Source: CAD feature listing. Evaluate the final solid. Frame: model axes, mm. Face numbers are marked on the shaded views. A direction names the side the tool comes from. Give positions to 0.01 mm unless a question says otherwise; leave off trailing zeros. Order: outer loops, then holes, each group sorted by start corner. A loop starts at its lowest first (then second) coordinate and runs counter-clockwise, first axis right, second up. Notation, with made-up numbers: M 84.25,-21.5 L 130.25,-21.5 A22 cw 130.25,4.5 Z; hole C 73,70.25 d11. An arc over 180 degrees is marked long. Return JSON: item names as keys, results as strings.
Solid Edge part; units mm, degrees
sketch "Sketch1" plane through (0, 0, 0) normal (0, -1, 0) x (1, 0, 0)
  arc A0 (87.9904, -3.3394) -> (81.4545, -9.3797) centre (75, 4.1606) cw
  arc A1 (81.4545, -9.3797) -> (51.8166, -19.1606) centre (28.049, 102.6551) cw
  line L0 (-51.8166, -19.1606) -> (51.8166, -19.1606)
  arc A2 (-81.4545, -9.3797) -> (-51.8166, -19.1606) centre (-28.049, 102.6551) ccw
  arc A3 (-73.8916, 19.1195) -> (-81.4545, -9.3797) centre (-75, 4.1606) ccw
  arc A4 (73.8916, 19.1195) -> (-73.8916, 19.1195) centre (0, 1016.3858) cw
  arc A5 (73.8916, 19.1195) -> (89.9997, 4.062) centre (75, 4.1606) cw
  arc A6 (87.9904, -3.3394) -> (89.9997, 4.062) centre (75, 4.1606) ccw
extrude "Protrusion1" add sketch "Sketch1" along normal mid plane 10
sketch "Sketch2" plane through (0, 0, 0) normal (0, -1, 0) x (1, 0, 0)
  circle A0 centre (-75, 4.1606) radius 12.5
  circle A1 centre (-38.1427, -9.4726) radius 7.5
  circle A2 centre (-13.3438, -9.4726) radius 7.5
  circle A3 centre (13.3438, -9.4726) radius 7.5
  circle A4 centre (38.1427, -9.4726) radius 7.5
  circle A5 centre (75, 4.1606) radius 12.5
extrude "ExtrudedProtrusion_2" add sketch "Sketch2" along normal blind 10
sketch "Sketch3" plane through (-75, -10, 4.1606) normal (0, -1, 0) x (1, 0, 0)
  arc A0 (162.5, 0) -> (137.5, 0) centre (150, 0) ccw
  line L0 (12.5, 0) -> (137.5, 0)
  arc A1 (-12.5, 0) -> (12.5, 0) centre (0, 0) cw
  line L1 (-12.5, 0) -> (-18.0005, 0)
  line L2 (-18.0005, 0) -> (-4.7328, 20)
  line L3 (0, 20) -> (-4.7328, 20)
  line L4 (150, 20) -> (0, 20)
  line L5 (150, 20) -> (154.7328, 20)
  line L6 (168.0005, 0) -> (154.7328, 20)
  line L7 (162.5, 0) -> (168.0005, 0)
extrude "Protrusion2" add sketch "Sketch3" against normal up to vertex (15 mm away)
sketch "Sketch4" plane through (-75, -10, 4.1606) normal (0, -1, 0) x (1, 0, 0)
  line L0 (0, 0) -> (150, 0)
  line L1 (150, 0) -> (168.0005, 0)
  line L2 (168.0005, 0) -> (154.7328, 20)
  line L3 (150, 20) -> (154.7328, 20)
  line L4 (150, 20) -> (0, 20)
  line L5 (0, 20) -> (-4.7328, 20)
  line L6 (-18.0005, 0) -> (-4.7328, 20)
  line L7 (0, 0) -> (-18.0005, 0)
extrude "ExtrudedCutout_2" cut sketch "Sketch4" against normal blind 2
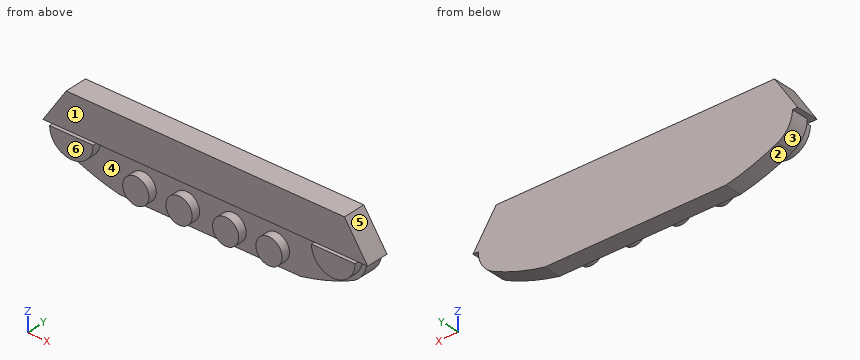
1. First-contact query: pin 1 (0.6 mm diameter, centred on x = -73.5, y = -8.5, fed in from +Z); pin 2 (8 mm diameter, centred on x = -42.5, z = 1.5, fed in from -Y); pin 3 (4.5 mm diameter, centred on x = 89.5, y = -1, fed in from -Z). Flat tips, straight axial feed; report the tip coordinate or a pass-through.
Evaluation:
{"pin 1": "stops at z = 4.16", "pin 2": "stops at y = -8", "pin 3": "stops at z = -4.5"}
2. Set-up query: the marked faces 1 and 2. Return all of +Z, -Z, +X, -X, +Y, -Y with unobstructed straight access to the full face (end or side cutting, diameter ignored); none if empty.
Evaluation:
{"face 1": "+Z, +X, -X, -Y", "face 2": "-Z, -X, +Y, -Y"}
3. Draft query along X for the marked faces 3, 4, 5 and 6. Return one class per face: pulls with the +X half, pulls with the -X half, needs draft (parallel to the pull), parting line crosses it, or undercut.
Evaluation:
{"face 3": "pulls with the -X half", "face 4": "undercut", "face 5": "pulls with the +X half", "face 6": "needs draft"}
4. Section query D-D (x = -74). Return loops of the section in (y, z), then the cut area to 3 significant figures.
Evaluation:
{"outline": "M -10,-8.3 L -5,-8.3 L -5,-12.64 L 5,-12.64 L 5,24.16 L -8,24.16 L -8,4.16 L -10,4.16 Z", "area": "490 mm^2"}
5. Section query B-B (x = -1). Return loops of the section in (y, z).
Evaluation:
{"outline": "M -8,4.16 L -5,4.16 L -5,-19.16 L 5,-19.16 L 5,24.16 L -8,24.16 Z"}
6. Section query C-C (z = -12). Return loops of the section in (x, y).
Evaluation:
{"outline": "M -75.57,-5 L -45.2,-5 L -45.2,-10 L -31.08,-10 L -31.08,-5 L -20.41,-5 L -20.41,-10 L -6.28,-10 L -6.28,-5 L 6.28,-5 L 6.28,-10 L 20.41,-10 L 20.41,-5 L 31.08,-5 L 31.08,-10 L 45.2,-10 L 45.2,-5 L 75.57,-5 L 75.57,5 L -75.57,5 Z"}
7. Section query A-A (y = -2.5). Return loops of the section in (x, z), then the cut area to 3 significant figures.
Evaluation:
{"outline": "M -93,4.16 L -90,4.16 A15 ccw -81.45,-9.38 A124.11 ccw -51.82,-19.16 L 51.82,-19.16 A124.11 ccw 81.45,-9.38 A15 ccw 90,4.16 L 93,4.16 L 79.73,24.16 L -79.73,24.16 Z", "area": "7,170 mm^2"}
8. Ray query, probe 1 along X at (y, z) = (-5.5, -10); probe 2 along Y at (x, z) = (86, 5.5); probe 3 along Y at (x, z) = (-5.5, -11). Return the intervals inside material, ascending.
Evaluation:
{"probe 1": "x = -45.62 to -30.66, -20.83 to -5.86, 5.86 to 20.83, 30.66 to 45.62", "probe 2": "y = -8 to 5", "probe 3": "y = -5 to 5"}
